For this review, take the finished solid that the model builds, in its own axes (mm). A direction names the side the tool comes from. Coordinates: 2 decimals unless noted, no trailing zeros. Write each loop counter-clockwise with the first axis right and the second up, starting at its lowest first coordinate (ties: lowest second). Pieces come first, ordered by that corner, then holes.
```python
from build123d import *

# Parameters (mm, degrees)
SKETCH1_R           = 3.25
SKETCH1_R_2         = 1.1811
SKETCH1_W           = 15
SKETCH1_H           = 6.858
BOSS_EXTRUDE1_DEPTH = 6.92


with BuildPart() as part:
    # Sketch1 → Boss-Extrude1 (new body)
    with BuildSketch(Plane.XY):
        with BuildLine():
            Line((54.449901472, -1.5), (93.949901472, -1.5))
            ThreePointArc((93.949901472, -1.5), (94.303454863, -1.353553391), (94.449901472, -1))
            Line((94.449901472, -1), (94.449901472, 12.686692025))
            Line((94.449901472, 12.686692025), (89.243377961, 47.938332641))
            ThreePointArc((89.243377961, 47.938332641), (88.235803145, 49.771012761), (86.275573302, 50.5))
            Line((86.275573302, 50.5), (83.280158812, 50.5))
            ThreePointArc((83.280158812, 50.5), (80.394529009, 51.308940401), (78.349901472, 53.5))
            Line((78.349901472, 53.5), (75.349901472, 53.5))
            Line((75.349901472, 53.5), (75.349901472, 60.26))
            Line((75.349901472, 60.26), (81.358592971, 60.26))
            ThreePointArc((81.358592971, 60.26), (82.095870308, 60.584409792), (82.354787669, 61.347155743))
            Line((82.354787669, 61.347155743), (78.044018988, 110.619467228))
            ThreePointArc((78.044018988, 110.619467228), (77.082205517, 112.56983201), (75.055434894, 113.358))
            Line((75.055434894, 113.358), (45.449901472, 113.358))
            Line((45.449901472, 113.358), (45.449901472, 60.26))
            Line((45.449901472, 60.26), (47.949901472, 60.26))
            Line((47.949901472, 60.26), (47.949901472, 53.5))
            Line((47.949901472, 53.5), (44.949901472, 53.5))
            ThreePointArc((44.949901472, 53.5), (44.596348081, 53.353553391), (44.449901472, 53))
            Line((44.449901472, 53), (44.449901472, 8.5))
            ThreePointArc((44.449901472, 8.5), (47.37883366, 1.428932188), (54.449901472, -1.5))
        make_face()
        with Locations((60.199901472, 47.5)):
            Circle(SKETCH1_R, mode=Mode.SUBTRACT)
        with Locations((60.199901472, 7.5)):
            Circle(SKETCH1_R, mode=Mode.SUBTRACT)
        with Locations((81.602701472, 3.5)):
            Circle(SKETCH1_R_2, mode=Mode.SUBTRACT)
        with Locations((90.949901472, 3.5)):
            Circle(SKETCH1_R_2, mode=Mode.SUBTRACT)
        with BuildLine():
            Line((72.399901472, 63.25), (69.999901472, 63.25))
            ThreePointArc((69.999901472, 63.25), (69.249901472, 64), (69.999901472, 64.75))
            Line((69.999901472, 64.75), (72.399901472, 64.75))
            ThreePointArc((72.399901472, 64.75), (73.149901472, 64), (72.399901472, 63.25))
        make_face(mode=Mode.SUBTRACT)
        with BuildLine():
            Line((72.399901472, 70.25), (69.999901472, 70.25))
            ThreePointArc((69.999901472, 70.25), (69.249901472, 71), (69.999901472, 71.75))
            Line((69.999901472, 71.75), (72.399901472, 71.75))
            ThreePointArc((72.399901472, 71.75), (73.149901472, 71), (72.399901472, 70.25))
        make_face(mode=Mode.SUBTRACT)
        with BuildLine():
            Line((60.174901472, 77.5), (60.174901472, 85.5))
            ThreePointArc((60.174901472, 85.5), (61.949901472, 87.275), (63.724901472, 85.5))
            Line((63.724901472, 85.5), (63.724901472, 77.5))
            ThreePointArc((63.724901472, 77.5), (61.949901472, 75.725), (60.174901472, 77.5))
        make_face(mode=Mode.SUBTRACT)
        with Locations((65.533922881, 106.929)):
            Rectangle(SKETCH1_W, SKETCH1_H, mode=Mode.SUBTRACT)
    extrude(amount=BOSS_EXTRUDE1_DEPTH)


solid = part.part
```
1) Consider section B-B (y = 80.5). Give the boundary of the cut face in (x, z), then the cut area to 3 significant figures.
2) For L1, parallel to Y at x = 62.5, z = 0.75; L2, parallel to Y at x = 58.5, z = 5; L3, parallel to Y at x = 84, z = 2, list the stretches that pass through material, from the lowest coordinate up.
3) Tool access review of faces 1 (the face through (80.431, 51.287, 3.412)), 2 (the face through (47.95, 57, 3)), 3 (the face through (85, 50.5, 3)), 4 (the face through (61.989, 75.725, 3.412)): name each direction out of +Z, -Z, +X, -X, +Y, -Y from which nothing blocks a thin tool from reaching the whole face with its end or side.
4) Clearance check with flat-ended pins moving along their axes: P1, Ø2, axis at y = 81, z = 2.5, coming from the -X side; P2, Ø2, axis at y = 108.5, z = 4, coming from the +X side; P3, Ø6, axis at x = 60.2, y = 7.5, coming from the -Z side; P4, Ø3.5, axis at y = 57, z = 4.5, coming from the +X side. State where each tip first meets the part, or that it passes through.
5) Consider section C-C (z = 1.5). Count the separate pieces of the cut face and the enclosed holes in it, then the cut area to 3 significant figures.
6) The part is to be moulded in two halves that separate along Y. For faces 5 (the face through (46, 53.5, 3)), 6 (the face through (64, 44, 0)), 7 (the face through (92.04, 3.05, 3.41)), 8 (the face through (88.26, 49.75, 3.41)), say which applies: pulls with the +Y half, pulls with the -Y half, needs draft (parallel to the pull), parting line crosses it, or undercut.
7) Consider section A-A (x = 66.5). Give the boundary of the cut face in (y, z).
8) Consider section D-D (x = 87.5). Give the boundary of the cut face in (y, z).
Results:
1. outline: (45.45, 0) - (60.17, 0) - (60.17, 6.92) - (45.45, 6.92) - close; (63.72, 0) - (80.68, 0) - (80.68, 6.92) - (63.72, 6.92) - close
1. area: 219 mm2
2. L1: y = -1.5 to 5.2, 9.8 to 45.2, 49.8 to 75.81, 87.19 to 103.5, 110.36 to 113.36
2. L2: y = -1.5 to 4.73, 10.27 to 44.73, 50.27 to 103.5, 110.36 to 113.36
2. L3: y = -1.5 to 50.5
3. face 1: +Z, -Z, +X
3. face 2: +Z, -Z, -X
3. face 3: +Z, -Z, +X, +Y
3. face 4: +Z, -Z
4. P1: stops at x = 45.45
4. P2: stops at x = 78.32
4. P3: passes through
4. P4: stops at x = 75.35
5. separate pieces: 1
5. enclosed holes: 8
5. area: 4,380 mm2
6. face 5: undercut
6. face 6: needs draft
6. face 7: undercut
6. face 8: pulls with the +Y half
7. outline: (-1.5, 0) - (103.5, 0) - (103.5, 6.92) - (-1.5, 6.92) - close; (110.36, 0) - (113.36, 0) - (113.36, 6.92) - (110.36, 6.92) - close
8. outline: (-1.5, 0) - (50.24, 0) - (50.24, 6.92) - (-1.5, 6.92) - close
